Autodesk Inventor part; units mm, degrees
ref_plane "YZ Plane" through (0, 0, 0) normal (1, 0, 0) x (0, 1, 0)
ref_plane "XZ Plane" through (0, 0, 0) normal (0, 1, 0) x (-1, 0, 0)
ref_plane "XY Plane" through (0, 0, 0) normal (0, 0, 1) x (1, 0, 0)
sketch "Sketch1" plane through (0, 0, 0) normal (0, 1, 0) x (-1, 0, 0)
  line L0 (0, 0) -> (-50.8, 0)
  line L1 (-50.8, 0) -> (-50.8, -63.5)
  line L2 (-50.8, -63.5) -> (0, -63.5)
  line L3 (0, -63.5) -> (0, 0)
  line L4 (-50.8, -63.5) -> (-50.8, -38.1)
  line L5 (-50.8, -38.1) -> (-25.4, -38.1)
  line L6 (-25.4, -38.1) -> (-25.4, 0)
  circle A0 centre (-25.4, -50.8) radius 2.0638
  line L7 (-50.8, -50.8) -> (0, -50.8) construction
  circle A1 centre (-38.1, -50.8) radius 2.0637
  circle A2 centre (-12.7, -50.8) radius 2.0637
  line L8 (-12.7, -63.5) -> (-12.7, 0) construction
  circle A3 centre (-12.7, -25.4) radius 2.0638
  circle A4 centre (-12.7, -12.7) radius 2.0638
  dimension "d22" = 50.8
  dimension "d23" = 63.5
  dimension "d24" = 25.4
  dimension "d25" = 25.4
  dimension "d26" = 4.1275
  dimension "d27" = 4.1275
  dimension "d28" = 12.7
  dimension "d29" = 4.1275
  dimension "d30" = 12.7
  dimension "d31" = 4.1275
  dimension "d32" = 25.4
  dimension "d33" = 4.1275
  dimension "d34" = 12.7
extrude "Extrusion1" add sketch "Sketch1" along normal blind 3.175 contours L3 L2 L1 L5 L6 L0
fillet "Fillet1" radius 6.35 5 edges at (50.8, 1.5875, -38.1) (25.4, 1.5875, 0) (0, 1.5875, 0) (0, 1.5875, -63.5) (50.8, 1.5875, -63.5)
properties part number "fram_support_gusset"
Input: part model. Units: mm. Frame: model coordinates. A direction names the side the tool comes from. Coordinates: 2 decimals unless noted, no trailing zeros. Order: outer loops, then holes, each group sorted by start corner. A loop starts at its lowest first (then second) coordinate and runs counter-clockwise, first axis right, second up. Notation, with made-up numbers: (-7.5, 59) - (2.5, 59) arc R21 cw to (2.5, 93) - close; hole circle Ø7 at (-24, 37.5). An arc over 180 degrees is marked (long way). Put each result on its own line as item: value.
1. Draft query along X for faces 1 (the face through (25.4, 2, -22)), 2 (the face through (14.338, 1.565, -11.444)), 3 (the face through (20, 3.175, -38)), 4 (the face through (14.338, 1.565, -49.544)). Return one class per face: pulls with the +X half, pulls with the -X half, needs draft (parallel to the pull), parting line crosses it, or undercut.
Report:
face 1: pulls with the +X half
face 2: undercut
face 3: needs draft
face 4: undercut
2. Line query: line 1 along Z through (x, y) = (12.7, 1.85); line 2 along Z through (x, y) = (38.1, 0.85); line 3 along Z through (x, y) = (14.5, 2.5). Output: solid intervals per line, ascending.
Report:
line 1: z = -63.5 to -52.86, -48.74 to -27.46, -23.34 to -14.76, -10.64 to 0
line 2: z = -63.5 to -52.86, -48.74 to -38.1
line 3: z = -63.5 to -51.81, -49.79 to -26.41, -24.39 to -13.71, -11.69 to 0
3. Cut plane C-C on x = 38.1. Return the cut outline in (y, z) (3 decimals), then the cut area to 3 significant figures.
Report:
outline: (0, -63.5) - (3.175, -63.5) - (3.175, -52.864) - (0, -52.864) - close; (0, -48.736) - (3.175, -48.736) - (3.175, -38.1) - (0, -38.1) - close
area: 67.5 mm2
4. Contact query for flat-ended pins moving along their axis: pin 1 Ø6.5 at (x, z) = (38.1, -50.8) entering from -Y; pin 2 Ø1.5 at (y, z) = (1, -27.5) entering from +X; pin 3 Ø2.5 at (x, z) = (12.7, -12.7) entering from +Y. Output: stop coordinate, or through.
Report:
pin 1: stops at y = 0
pin 2: stops at x = 25.4
pin 3: passes through
5. Cut plane A-A on z = -50.8. Return the cut outline in (x, y) (3 decimals).
Report:
outline: (0, 0) - (10.636, 0) - (10.636, 3.175) - (0, 3.175) - close; (14.764, 0) - (23.336, 0) - (23.336, 3.175) - (14.764, 3.175) - close; (27.464, 0) - (36.036, 0) - (36.036, 3.175) - (27.464, 3.175) - close; (40.164, 0) - (50.8, 0) - (50.8, 3.175) - (40.164, 3.175) - close
6. Reachability of faces 5 (the face through (1.91, 1.61, -61.69)), 6 (the face through (35, 2, -38.1)) from +Z, -Z, +X, -X, +Y, -Y: full face, straight path, thin tool, end or side. Return the list, or none.
Report:
face 5: -Z, -X, +Y, -Y
face 6: +Z, +X, +Y, -Y
7. Cut plane D-D on z = -12.7. Return the cut outline in (x, y) (3 decimals).
Report:
outline: (0, 0) - (10.636, 0) - (10.636, 3.175) - (0, 3.175) - close; (14.764, 0) - (25.4, 0) - (25.4, 3.175) - (14.764, 3.175) - close
8. Cut plane B-B on y = 1.85. Return the cut outline in (x, z).
Report:
outline: (0, -57.15) arc R6.35 ccw to (6.35, -63.5) - (44.45, -63.5) arc R6.35 ccw to (50.8, -57.15) - (50.8, -44.45) arc R6.35 ccw to (44.45, -38.1) - (25.4, -38.1) - (25.4, -6.35) arc R6.35 ccw to (19.05, 0) - (6.35, 0) arc R6.35 ccw to (0, -6.35) - close; hole circle Ø4.13 at (12.7, -50.8); hole circle Ø4.13 at (12.7, -25.4); hole circle Ø4.13 at (12.7, -12.7); hole circle Ø4.13 at (25.4, -50.8); hole circle Ø4.13 at (38.1, -50.8)
